```python
from build123d import *

# Parameters (mm, degrees)
SKETCH1_W           = 18
SKETCH1_H           = 32
BOSS_EXTRUDE1_DEPTH = 3
SKETCH2_R           = 1.5
CUT_EXTRUDE2_DEPTH  = 3


with BuildPart() as part:
    # Sketch1 → Boss-Extrude1 (new body)
    with BuildSketch(Plane(origin=(0, 0, 0), x_dir=(0, 0, -1), z_dir=(1, 0, 0))):
        Rectangle(SKETCH1_W, SKETCH1_H)
    extrude(amount=BOSS_EXTRUDE1_DEPTH)

    # Sketch2 → Cut-Extrude2 (cut)
    with BuildSketch(Plane(origin=(3, 0, 0), x_dir=(0, 0, -1), z_dir=(1, 0, 0))):
        with BuildLine():
            ThreePointArc((8, 16), (8.707106781, 15.707106781), (9, 15))
            Line((9, 15), (9, 16))
            Line((9, 16), (8, 16))
        make_face()
        with BuildLine():
            ThreePointArc((-9, 15), (-8.707106781, 15.707106781), (-8, 16))
            Line((-8, 16), (-9, 16))
            Line((-9, 16), (-9, 15))
        make_face()
        with BuildLine():
            Line((-6, -16), (-5, -16))
            ThreePointArc((-5, -16), (-5.707106781, -15.707106781), (-6, -15))
            Line((-6, -15), (-6, 11))
            Line((-6, 11), (-9, 11))
            Line((-9, 11), (-9, -16))
            Line((-9, -16), (-6, -16))
        make_face()
        with BuildLine():
            Line((6, 11), (6, -15))
            ThreePointArc((6, -15), (5.707106781, -15.707106781), (5, -16))
            Line((5, -16), (6, -16))
            Line((6, -16), (9, -16))
            Line((9, -16), (9, 11))
            Line((9, 11), (6, 11))
        make_face()
        with Locations((0, 5.5)):
            Circle(SKETCH2_R)
        with Locations((0, -12)):
            Circle(SKETCH2_R)
    extrude(amount=-CUT_EXTRUDE2_DEPTH, mode=Mode.SUBTRACT)


solid = part.part
```
The model under review builds one solid part; all positions refer to its coordinate system, in mm. A direction names the side the tool comes from. Round coordinates to 2 decimals unless told otherwise and drop trailing zeros. Order: outer loops, then holes, each group sorted by start corner. A loop starts at its lowest first (then second) coordinate and runs counter-clockwise, first axis right, second up. Notation, with made-up numbers: M 77.25,25 L 125.25,25 A29 ccw 125.25,54 Z; hole C -20.5,48.5 d1. An arc over 180 degrees is marked long. Use a Markdown table: item, result.
1) Consider section C-C (x = 1.65). Write out the cut boundary in (y, z), then the cut area to 3 significant figures.
Report:
| item | result |
|---|---|
| outline | M -16,-5 A1 ccw -15,-6 L 11,-6 L 11,-9 L 15,-9 A1 ccw 16,-8 L 16,8 A1 ccw 15,9 L 11,9 L 11,6 L -15,6 A1 ccw -16,5 Z; hole C -12,0 d3; hole C 5.5,0 d3 |
| area | 399 mm^2 |
2) Tool access review of faces 5 (the face through (2, -2, 6)), 6 (the face through (1, -16, 0)), 7 (the face through (2, 11, -8)): name each direction out of +Z, -Z, +X, -X, +Y, -Y from which nothing blocks a thin tool from reaching the whole face with its end or side.
Report:
| item | result |
|---|---|
| face 5 | +Z, +X, -X, -Y |
| face 6 | +Z, -Z, +X, -X, -Y |
| face 7 | -Z, +X, -X, -Y |
3) Draft analysis for pull direction Y (two halves, no side actions). For faces 1 (the face through (1, 16, 0)), 2 (the face through (0, 0, 0)), 3 (the face through (2, 4, 0)), 4 (the face through (2, 11, 7)), state which applies: released by +Y, released by -Y, zero draft, split by the parting line, or undercut.
Report:
| item | result |
|---|---|
| face 1 | released by +Y |
| face 2 | zero draft |
| face 3 | undercut |
| face 4 | released by -Y |
4) Consider section A-A (y = 5.5). Write out the cut boundary in (x, z), then the cut area to 3 significant figures.
Report:
| item | result |
|---|---|
| outline | M 0,-6 L 3,-6 L 3,-1.5 L 0,-1.5 Z; M 0,1.5 L 3,1.5 L 3,6 L 0,6 Z |
| area | 27.0 mm^2 |
5) Consider section B-B (z = 0). Write out the cut boundary in (x, y).
Report:
| item | result |
|---|---|
| outline | M 0,-16 L 3,-16 L 3,-13.5 L 0,-13.5 Z; M 0,-10.5 L 3,-10.5 L 3,4 L 0,4 Z; M 0,7 L 3,7 L 3,16 L 0,16 Z |
6) Wall thickness on line 1 along Y through (x, z) = (2.2, 0); line 2 along Y through (x, z) = (1.1, 0.5); line 3 along Z through (x, y) = (1.2, -6.5): over which ranges is each line inside the solid? List them lowest first. Write a range as [from, to].
Report:
| item | result |
|---|---|
| line 1 | [-16, -13.5], [-10.5, 4], [7, 16] |
| line 2 | [-16, -13.41], [-10.59, 4.09], [6.91, 16] |
| line 3 | [-6, 6] |
7) Consider section D-D (z = -6.75). Write out the cut boundary in (x, y).
Report:
| item | result |
|---|---|
| outline | M 0,11 L 3,11 L 3,16 L 0,16 Z |
8) Insertion check: pin 1 (0.9 mm diameter, centred on x = 2, y = 0.5, fed in from -Z); pin 2 (1 mm diameter, centred on x = 2, y = 2, fed in from +Z); pin 3 (1.5 mm diameter, centred on x = 1.5, z = 7.5, fed in from -Y). Each pin has a flat end and moves straight along its axis. Give the tip position at first contact, or say it passes through.
Report:
| item | result |
|---|---|
| pin 1 | z = -6 |
| pin 2 | z = 6 |
| pin 3 | y = 11 |
